```python
from build123d import *

# Parameters (mm, degrees)
BOSS_EXTRUDE1_DEPTH = 13
SKETCH2_W           = 12.000442616
SKETCH2_H           = 1
BOSS_EXTRUDE2_DEPTH = 2.25
CUT_EXTRUDE2_REACH  = 25.453
SKETCH5_W           = 4
SKETCH5_H           = 2.25
SKETCH6_W           = 7
SKETCH6_H           = 2
BOSS_EXTRUDE4_DEPTH = 2.25
SKETCH4_W           = 5
SKETCH4_H           = 1
CUT_EXTRUDE1_DEPTH  = 21.076474399
SKETCH7_W           = 5.25
SKETCH7_H           = 4.75
SKETCH7_W_2         = 5.45
BOSS_EXTRUDE5_DEPTH = 1.5
FILLET5_R           = 1
FILLET6_R           = 1


with BuildPart() as part:
    # Sketch1 → Boss-Extrude1 (new body)
    with BuildSketch(Plane.XY):
        Polygon((-7, -13.603853288), (-1.75, -13.603853288), (-1.75, -12.603853288), (1.75, -12.603853288), (1.75, -13.603853288), (7, -13.603853288), (7, -12.103853288), (7, -9.853853288), (6.000442616, -9.853853288), (6.000442616, -12.103853288), (-6, -12.103853288), (-6, -9.853853288), (-7, -9.853853288), (-7, -12.103853288), align=None)
    extrude(amount=BOSS_EXTRUDE1_DEPTH)

    # Sketch2 → Boss-Extrude2 (add)
    with BuildSketch(Plane(origin=(0, -12.103853288, 0), x_dir=(1, 0, 0), z_dir=(0, 1, 0))):
        with Locations((0.000221308, -0.5)):
            Rectangle(SKETCH2_W, SKETCH2_H)
        with Locations((0.000221308, -12.5)):
            Rectangle(SKETCH2_W, SKETCH2_H)
    extrude(amount=BOSS_EXTRUDE2_DEPTH)

    # Cut-Extrude2: up to this face of the body (flat: up to its plane)
    cut_extrude2_end = Plane(part.part.faces().sort_by_distance((7, -11.728853288, 6.5))[0])
    # Sketch5 → Cut-Extrude2 (cut, up to the picked face)
    with BuildSketch(Plane.ZY.offset(7), mode=Mode.PRIVATE) as cut_extrude2_sk1:
        with Locations((6.5, -10.978853288)):
            Rectangle(SKETCH5_W, SKETCH5_H)
    cut_extrude2_tool1 = split(extrude(cut_extrude2_sk1.sketch, amount=-CUT_EXTRUDE2_REACH, mode=Mode.PRIVATE), bisect_by=cut_extrude2_end, keep=Keep.BOTH, mode=Mode.PRIVATE)
    add(cut_extrude2_tool1.solids().sort_by(Axis((-7, -10.978853, 6.5), (1, 0, 0)))[0], mode=Mode.SUBTRACT)

    # Sketch6 → Boss-Extrude4 (add)
    with BuildSketch(Plane(origin=(0, -12.103853288, 0), x_dir=(1, 0, 0), z_dir=(0, 1, 0))):
        with Locations((0, -6.5)):
            Rectangle(SKETCH6_W, SKETCH6_H)
    extrude(amount=BOSS_EXTRUDE4_DEPTH)

    # Sketch4 → Cut-Extrude1 (cut, through all)
    with BuildSketch(Plane(origin=(0, 0, 0), x_dir=(-1, 0, 0), z_dir=(0, 0, -1))):
        with Locations((0, -10.353853288)):
            Rectangle(SKETCH4_W, SKETCH4_H)
    extrude(amount=-CUT_EXTRUDE1_DEPTH, mode=Mode.SUBTRACT)

    # Sketch7 → Boss-Extrude5 (add)
    with BuildSketch(Plane(origin=(0, 0, 0), x_dir=(-1, 0, 0), z_dir=(0, 0, -1))):
        with Locations((4.375, -11.228853288)):
            Rectangle(SKETCH7_W, SKETCH7_H)
        with Locations((-4.275, -11.228853288)):
            Rectangle(SKETCH7_W_2, SKETCH7_H)
    extrude(amount=BOSS_EXTRUDE5_DEPTH)

    # Fillet5
    fillet5_edges = [part.edges().sort_by_distance(p)[0] for p in [
        (4.375, -13.603853288, 13),
        (-4.375, -13.603853288, -1.5),
        (-4.375, -13.603853288, 13),
        (-7, -13.603853288, 5.75),
        (7, -13.603853288, 5.75),
        (4.275, -13.603853288, -1.5),
    ]]
    fillet(fillet5_edges, radius=FILLET5_R)

    # Fillet6
    fillet6_edges = [part.edges().sort_by_distance(p)[0] for p in [
        (-7, -8.853853288, -0.75),
        (7, -8.853853288, -0.75),
        (-4.375, -8.853853288, -1.5),
        (4.275, -8.853853288, -1.5),
    ]]
    fillet(fillet6_edges, radius=FILLET6_R)


solid = part.part
```
Could you check a few things on this model? Use its own coordinates, in mm. A direction names the side the tool comes from. Coordinates: 2 decimals unless noted, no trailing zeros. Order: outer loops, then holes, each group sorted by start corner. A loop starts at its lowest first (then second) coordinate and runs counter-clockwise, first axis right, second up. Notation, with made-up numbers: M 45,25 L 67,25 A21 ccw 67,32 Z; hole C 59.25,45 d3. An arc over 180 degrees is marked long. Use one line per item in the form item = value. Start each with the question number.
1. For pin 1 (0.8 mm diameter, centred on y = -13, z = 8, fed in from -X); pin 2 (6 mm diameter, centred on x = 1.5, z = 7.5, fed in from +Y); pin 3 (2 mm diameter, centred on x = 4.5, z = 10, fed in from +Y); pin 4 (0.8 mm diameter, centred on y = -10, z = 6, fed in from -X), each with a flat end and sliding along its axis, tell me the tip position at first contact or that it passes through.
2. Suppose I cut it at C-C on z = 5. Write out the boundary of the cut face in (x, y), then the cut area to 3 significant figures.
3. Suppose I cut it at D-D on y = -13.1. Write out the boundary of the cut face in (x, z), then the cut area to 3 significant figures.
4. On a 3-axis mill with a long thin cutter (end or side, diameter ignored), from which of +Z, -Z, +X, -X, +Y, -Y can I reach the whole of each face in a straight line? I mean faces 4 (the flat face through (-6.5, -11, 8.5)), 5 (the flat face through (0, -10.854, 0.5)), 6 (the flat face through (6, -11, 3)). Say none if no direction works.
5. Suppose I cut it at B-B on x = -0.75. Write out the boundary of the cut face in (y, z).
6. Please list where these lines run through material, in increasing order: line 1 (Z direction, x = -2.75, y = -10.4); line 2 (Z direction, x = -5.25, y = -10.4); line 3 (X direction, y = -12, z = 11.75).
7. We'd pull the mould along Z, two halves only. Please class faces 1 (the flat face through (0, -10.854, 12.5)), 2 (the cylindrical face through (-4.41, -13.32, -1.2)), 3 (the flat face through (-6, -11, 3)): +Z half, -Z half, draft (parallel to the pull), parting line (faces both ways), or undercut.
8. Suppose I cut it at A-A on y = -11.45. Write out the boundary of the cut face in (x, z).
Geometry says:
q1.pin_1 = -7
q1.pin_2 = -9.85
q1.pin_3 = -12.1
q1.pin_4 = -3.5
q2.outline = M -7,-12.6 A1 ccw -6,-13.6 L -1.75,-13.6 L -1.75,-12.6 L 1.75,-12.6 L 1.75,-13.6 L 6,-13.6 A1 ccw 7,-12.6 L 7,-12.1 L -7,-12.1 Z
q2.area = 17.1 mm^2
q3.outline = M -6.87,-1.37 L -1.75,-1.37 L -1.75,12.87 L -6.87,12.87 Z; M 1.55,-1.37 L 6.87,-1.37 L 6.87,12.87 L 1.75,12.87 L 1.75,0 L 1.55,0 Z
q3.area = 146 mm^2
q4.face_4 = +X, -X, +Y
q4.face_5 = +Z, +Y
q4.face_6 = +Y
q5.outline = M -12.6,0 L -10.85,0 L -10.85,1 L -12.1,1 L -12.1,5.5 L -10.85,5.5 L -10.85,7.5 L -12.1,7.5 L -12.1,12 L -10.85,12 L -10.85,13 L -12.6,13 Z
q6.line_1 = -1.5 to 1, 5.5 to 7.5, 12 to 13
q6.line_2 = -1.5 to 1, 12 to 13
q6.line_3 = -7 to -6, 6 to 7
q7.face_1 = draft
q7.face_2 = -Z half
q7.face_3 = undercut
q8.outline = M -7,-1.5 L -1.75,-1.5 L -1.75,0 L 1.55,0 L 1.55,-1.5 L 7,-1.5 L 7,4.5 L 6,4.5 L 6,1 L -6,1 L -6,4.5 L -7,4.5 Z; M -7,8.5 L -6,8.5 L -6,12 L 6,12 L 6,8.5 L 7,8.5 L 7,13 L -7,13 Z; M -3.5,5.5 L 3.5,5.5 L 3.5,7.5 L -3.5,7.5 Z
